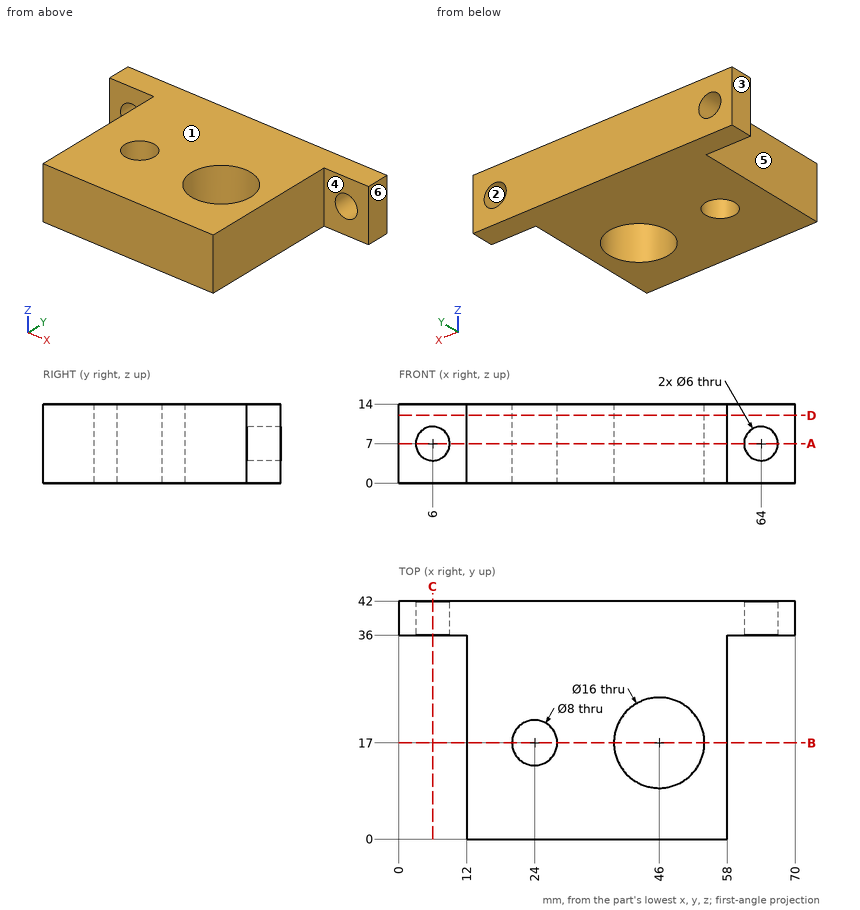
Geometry check sheet. Reference: drawing and pictorial views, mm from the part's lowest x, y, z. A direction names the side the tool comes from. Round coordinates to 2 decimals unless told otherwise and drop trailing zeros. Write each loop counter-clockwise with the first axis right and the second up, starting at its lowest first coordinate (ties: lowest second). Pieces come first, ordered by that corner, then holes. Notation, with made-up numbers: (-12.5, 60.25) -> (9.5, 60.25) arc R19 cw to (9.5, 86.25) -> close; hole circle Ø10 at (12.25, 30). An arc over 180 degrees is marked (long way). One line per question, with ' | ' between items. Start each with the question number.
1. Set-up check for the marked faces 4, 5 and 6: record each of +Z, -Z, +X, -X, +Y, -Y from which the full face is reachable in a straight line by a thin tool's end or side.
2. Sectioned sample at B-B, the plane y = 17. Record the cut outline in (x, z), then the cut area to 3 significant figures.
3. Release check for a two-part mould opening along X. For the marked faces 1, 2 and 3 record: +X half, -X half, draft (parallel to the pull), parting line (faces both ways), or undercut.
4. Sectioned sample at C-C, the plane x = 6. Record the cut outline in (y, z).
5. Sectioned sample at D-D, the plane z = 12. Record the cut outline in (x, y), then the cut area to 3 significant figures.
6. Depth check by flat-ended pin: pin 1 (12 mm diameter, centred on x = 56, y = 36.5, fed in from -Z); pin 2 (3.5 mm diameter, centred on x = 4, z = 9, fed in from -Y); pin 3 (4 mm diameter, centred on y = 17, z = 10.5, fed in from +X); pin 4 (5 mm diameter, centred on x = 6, z = 7, fed in from -Y). Enter the tip coordinate at first touch or a pass-through.
7. Sectioned sample at A-A, the plane z = 7. Record the cut outline in (x, y), then the cut area to 3 significant figures.
8. Scan lines: line 1 along Y through (x, z) = (24, 3.5); line 2 along X through (y, z) = (37.5, 5.25); line 3 along Z through (x, y) = (64, 39). Record each from-to range of solid material in increasing order. Write a range as from..to.
Taken from the geometry:
1) face 4: +Z, -Z, +X, -Y | face 5: +Z, -Z, -X, -Y | face 6: +Z, -Z, +X, +Y, -Y
2) outline: (12, 0) -> (20, 0) -> (20, 14) -> (12, 14) -> close; (28, 0) -> (38, 0) -> (38, 14) -> (28, 14) -> close; (54, 0) -> (58, 0) -> (58, 14) -> (54, 14) -> close | area: 308 mm^2
3) face 1: draft | face 2: undercut | face 3: -X half
4) outline: (36, 0) -> (42, 0) -> (42, 4) -> (36, 4) -> close; (36, 10) -> (42, 10) -> (42, 14) -> (36, 14) -> close
5) outline: (0, 36) -> (12, 36) -> (12, 0) -> (58, 0) -> (58, 36) -> (70, 36) -> (70, 42) -> (0, 42) -> close; hole circle Ø8 at (24, 17); hole circle Ø16 at (46, 17) | area: 1,820 mm^2
6) pin 1: stops at z = 0 | pin 2: stops at y = 36 | pin 3: stops at x = 58 | pin 4: passes through
7) outline: (0, 36) -> (3, 36) -> (3, 42) -> (0, 42) -> close; (9, 36) -> (12, 36) -> (12, 0) -> (58, 0) -> (58, 36) -> (61, 36) -> (61, 42) -> (9, 42) -> close; (67, 36) -> (70, 36) -> (70, 42) -> (67, 42) -> close; hole circle Ø8 at (24, 17); hole circle Ø16 at (46, 17) | area: 1,750 mm^2
8) line 1: y = 0..13, 21..42 | line 2: x = 0..3.56, 8.44..61.56, 66.44..70 | line 3: z = 0..4, 10..14
